Build history of the part. All positions in model axes, mm. A direction names the side the tool comes from. Give positions to 0.01 mm unless a question says otherwise; leave off trailing zeros. Loops run counter-clockwise (first coordinate to the right, second up) from the corner with the lowest first, then second, coordinate; pieces in that order, holes last.
1) Band-saw the part on B-B on x = 43.75. List the corners of the cut face in (y, z).
2) Two-plate mould, pull along X, no slides. Class faces 1 (the flat face through (56.972, 0, 0)), 2 (the flat face through (45.123, 13, -16)), 3 (the cylindrical face through (52.77, -8.26, -19.92)), 4 (the cylindrical face through (46.93, 19.81, -4.4)): +X half, -X half, draft (parallel to the pull), parting line (faces both ways), or undercut.
3) Wall check: line 1 (X direction, y = -14.5, z = 15.5); line 2 (Y direction, x = 54.5, z = -5); line 3 (Z direction, x = 42.25, y = 14.5). Give the ranges that are in metal, low to high.
4) Flat gauge pins, fed straight in: P1, Ø1, axis at x = 48, y = 7.5, coming from the -Z side; P2, Ø3, axis at x = 49.5, z = -14.5, coming from the -Y side; P3, Ø6, axis at x = 52.5, z = 9.5, coming from the +Y side; P4, Ø2, axis at y = -16.5, z = 14, coming from the +X side. Where does each tip first touch, or does it go through?
5) 3-axis set-ups, long thin cutter, end or side, ignore diameter. For faces 5 (the flat face through (48.679, 13, -16)), 6 (the cylindrical face through (40.92, -8.26, -19.92)): which of +Z, -Z, +X, -X, +Y, -Y reach the whole face in a straight line?
6) Band-saw the part on A-A on y = 17. List the corners of the cut face in (x, z), then the cut area to 3 significant figures.
7) Band-saw the part on C-C on z = -16. List the corners of the cut face in (x, y), then the cut area to 3 significant figures.
```python
from build123d import *

# Parameters (mm, degrees)
SKETCH8_R           = 21.5646
BOSS_EXTRUDE1_DEPTH = 20.1422
SKETCH9_W           = 3.556
SKETCH9_H           = 1.27


with BuildPart() as part:
    # Sketch8 → Boss-Extrude1 (new body)
    with BuildSketch(Plane(origin=(36.83, 0, 0), x_dir=(0, 0, -1), z_dir=(1, 0, 0))):
        Circle(SKETCH8_R)
    extrude(amount=BOSS_EXTRUDE1_DEPTH)

    # Sketch9 → O-Ring Groove 2-128ish (revolve, cut)
    with BuildSketch(Plane.XY, mode=Mode.PRIVATE) as o_ring_groove_2_128ish_sk:
        with Locations((46.9011, 20.9296)):
            Rectangle(SKETCH9_W, SKETCH9_H)
    revolve(o_ring_groove_2_128ish_sk.sketch.rotate(Axis((-14.406993702, 0, 0), (1, 0, 0)), 90), axis=Axis((-14.406993702, 0, 0), (1, 0, 0)), mode=Mode.SUBTRACT)


solid = part.part
```
Findings below:
1. outline: circle Ø43.13 at (0, 0)
2. face 1: +X half
2. face 2: undercut
2. face 3: draft
2. face 4: undercut
3. line 1: x = 36.83 to 45.12, 48.68 to 56.97
3. line 2: y = -20.98 to 20.98
3. line 3: z = -15.96 to 15.96
4. P1: stops at z = -19.05
4. P2: stops at y = -17.21
4. P3: stops at y = 20.56
4. P4: stops at x = 56.97
5. face 5: none
5. face 6: +X, -X
6. outline: (36.83, -13.27) - (45.12, -13.27) - (45.12, -11.08) - (48.68, -11.08) - (48.68, -13.27) - (56.97, -13.27) - (56.97, 13.27) - (48.68, 13.27) - (48.68, 11.08) - (45.12, 11.08) - (45.12, 13.27) - (36.83, 13.27) - close
6. area: 519 mm2
7. outline: (36.83, -14.46) - (45.12, -14.46) - (45.12, -12.48) - (48.68, -12.48) - (48.68, -14.46) - (56.97, -14.46) - (56.97, 14.46) - (48.68, 14.46) - (48.68, 12.48) - (45.12, 12.48) - (45.12, 14.46) - (36.83, 14.46) - close
7. area: 568 mm2
